Source: CAD feature listing. Evaluate the final solid. Frame: model axes, mm. Give positions to 0.01 mm unless a question says otherwise; leave off trailing zeros. Order: outer loops, then holes, each group sorted by start corner. A loop starts at its lowest first (then second) coordinate and runs counter-clockwise, first axis right, second up. Notation, with made-up numbers: (-10.75, -18) - (26.25, -18) arc R24 cw to (26.25, 17) - close; hole circle Ø4 at (48.5, -32). An arc over 180 degrees is marked (long way). Answer as CSV lines item,"result".
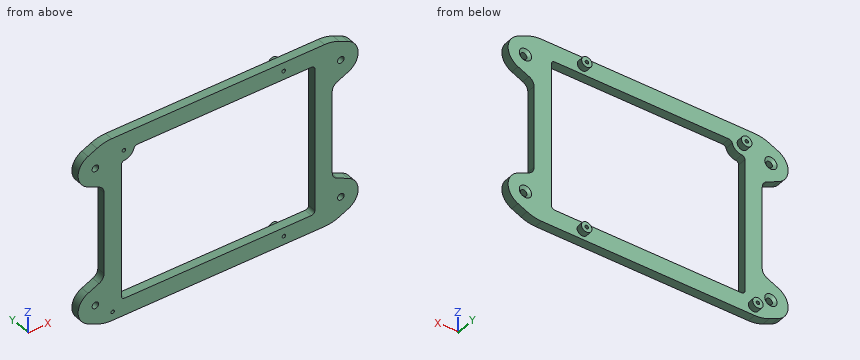
```python
from build123d import *

# Parameters (mm, degrees)
QUARTER_BASE_DEPTH                 = 5
CORNER_SCREW_EXPANSION_SKETCH_R    = 6.025
CORNER_SCREW_EXPANSION_DEPTH       = 5
STANDOFFS_EXTRUSION_SKETCH_R       = 3.025
STANDOFFS_EXTRUSION_DEPTH          = 3.5
SMOOTHIEBOARD_SCREW_HOLES_SKETCH_R = 1.025
SMOOTHIEBOARD_SCREW_HOLES_DEPTH    = 98.695404319
NO_6_MOUNTING_SCREWS_D             = 3.7973
NO_6_MOUNTING_SCREWS_CSINK_D       = 7.0866
NO_6_MOUNTING_SCREWS_CSINK_ANGLE   = 100
INSIDE_CORNER_FILLETS_R            = 2
OUTSIDE_CORNER_FILLETS_1_R         = 5
OUTSIDE_CORNER_FILLETS_2_R         = 20


with BuildPart() as part:
    # Quarter Base Sketch → Quarter Base (new body)
    with BuildSketch(Plane(origin=(0, 0, 0), x_dir=(1, 0, 0), z_dir=(0, 1, 0))):
        with BuildLine():
            Line((0, 53.955), (-66, 53.955))
            Line((-66, 53.955), (-75.226182617, 49.65276039))
            ThreePointArc((-75.226182617, 49.65276039), (-81, 40.58968252), (-75.226182617, 31.526604649))
            Line((-75.226182617, 31.526604649), (-66, 27.224365039))
            Line((-66, 27.224365039), (-66, 0))
            Line((-66, 0), (-56, 0))
            Line((-56, 0), (-56, 43.955))
            Line((-56, 43.955), (0, 43.955))
            Line((0, 43.955), (0, 53.955))
        make_face()
    extrude(amount=QUARTER_BASE_DEPTH)

    # Base Mirror 1: part across plane


with BuildPart() as part_1:
    add(part.part)
    add(part.part.mirror(Plane(origin=(-66, 5, 0), x_dir=(1, 0, 0), z_dir=(0, 0, -1))))

    # Base Mirror 2: part across plane


with BuildPart() as part_2:
    add(part_1.part)
    add(part_1.part.mirror(Plane(origin=(0, 5, -43.955), x_dir=(0, 0, 1), z_dir=(-1, 0, 0))))

    # Corner Screw Expansion Sketch → Corner Screw Expansion (add)
    with BuildSketch(Plane(origin=(0, 5, 0), x_dir=(1, 0, 0), z_dir=(0, 1, 0))):
        with Locations((-54.523, -43.876)):
            Circle(CORNER_SCREW_EXPANSION_SKETCH_R)
    extrude(amount=-CORNER_SCREW_EXPANSION_DEPTH)

    # Standoffs Extrusion Sketch → Standoffs Extrusion (add)
    with BuildSketch(Plane(origin=(0, 5, 0), x_dir=(1, 0, 0), z_dir=(0, 1, 0))):
        with Locations(Location((-61, 48.955, 0), (0, 0, 270))):
            Circle(STANDOFFS_EXTRUSION_SKETCH_R)
        with Locations(Location((-54.523, -43.876, 0), (0, 0, 270))):
            Circle(STANDOFFS_EXTRUSION_SKETCH_R)
        with Locations(Location((37.933, -48.955, 0), (0, 0, 270))):
            Circle(STANDOFFS_EXTRUSION_SKETCH_R)
        with Locations(Location((38.06, 48.955, 0), (0, 0, 270))):
            Circle(STANDOFFS_EXTRUSION_SKETCH_R)
    extrude(amount=STANDOFFS_EXTRUSION_DEPTH)

    # Smoothieboard Screw Holes Sketch → Smoothieboard Screw Holes (cut, through all)
    with BuildSketch(Plane(origin=(0, 8.5, 0), x_dir=(1, 0, 0), z_dir=(0, 1, 0))):
        with Locations(Location((-54.523, -43.876, 0), (0, 0, 270))):
            Circle(SMOOTHIEBOARD_SCREW_HOLES_SKETCH_R)
        with Locations(Location((37.933, -48.955, 0), (0, 0, 270))):
            Circle(SMOOTHIEBOARD_SCREW_HOLES_SKETCH_R)
        with Locations(Location((38.06, 48.955, 0), (0, 0, 270))):
            Circle(SMOOTHIEBOARD_SCREW_HOLES_SKETCH_R)
        with Locations(Location((-61, 48.955, 0), (0, 0, 270))):
            Circle(SMOOTHIEBOARD_SCREW_HOLES_SKETCH_R)
    extrude(amount=-SMOOTHIEBOARD_SCREW_HOLES_DEPTH, mode=Mode.SUBTRACT)

    # No. 6 Mounting Screws (through all)
    with Locations(Plane(origin=(-71, 5, -40.58968252), x_dir=(0, 0, 1), z_dir=(0, 1, 0))):
        with Locations((0, 0), (81.17936504, 0), (81.17936504, 142), (0, 142)):
            CounterSinkHole(NO_6_MOUNTING_SCREWS_D / 2, NO_6_MOUNTING_SCREWS_CSINK_D / 2, counter_sink_angle=NO_6_MOUNTING_SCREWS_CSINK_ANGLE)

    # Inside Corner Fillets
    inside_corner_fillets_edges = [part_2.edges().sort_by_distance(p)[0] for p in [
        (-56, 2.5, -43.955),
        (56, 2.5, -43.955),
        (56, 2.5, 43.955),
        (-48.498517948, 2.5, 43.955),
        (-56, 2.5, 38.034844635),
    ]]
    fillet(inside_corner_fillets_edges, radius=INSIDE_CORNER_FILLETS_R)

    # Outside Corner Fillets 1
    outside_corner_fillets_1_edges = [part_2.edges().sort_by_distance(p)[0] for p in [
        (-66, 2.5, -27.224365039),
        (-66, 2.5, 27.224365039),
        (66, 2.5, -27.224365039),
        (66, 2.5, 27.224365039),
    ]]
    fillet(outside_corner_fillets_1_edges, radius=OUTSIDE_CORNER_FILLETS_1_R)

    # Outside Corner Fillets 2
    outside_corner_fillets_2_edges = [part_2.edges().sort_by_distance(p)[0] for p in [
        (-66, 2.5, -53.955),
        (-66, 2.5, 53.955),
        (66, 2.5, -53.955),
        (66, 2.5, 53.955),
    ]]
    fillet(outside_corner_fillets_2_edges, radius=OUTSIDE_CORNER_FILLETS_2_R)


solid = part_2.part
```
(1) Ray query, line 1 (X direction, y = 1.75, z = 23.5); line 2 (Z direction, x = 71, y = 2.5); line 3 (Z direction, x = -2, y = 3) (3 decimals). Return the intervals inside material, ascending. Write a range as from..to.
Completed:
line 1,"-66..-56, 56..66"
line 2,"-51.62..-42.49, -38.69..-29.56, 29.56..38.69, 42.49..51.62"
line 3,"-53.955..-43.955, 43.955..53.955"
(2) Cut plane A-A (x = -30). Return loops of the section in (y, z) (3 decimals).
Completed:
outline,"(0, -53.955) - (5, -53.955) - (5, -43.955) - (0, -43.955) - close; (0, 43.955) - (5, 43.955) - (5, 53.955) - (0, 53.955) - close"
(3) Contact query for flat-ended pins moving along their axis: pin 1 (2.5 mm diameter, centred on x = -54.523, z = 43.876, fed in from +Y); pin 2 (1.2 mm diameter, centred on x = -61, z = -48.955, fed in from -Y); pin 3 (4.5 mm diameter, centred on x = 71, z = 40.59, fed in from +Y); pin 4 (1.5 mm diameter, centred on y = 2.5, z = 4.5, fed in from +X). Output: stop coordinate, or through.
Completed:
pin 1,"y = 8.5"
pin 2,"through"
pin 3,"y = 3.92"
pin 4,"x = 66"
(4) Cut plane B-B (z = 12.5). Return loops of the section in (x, y), then the cut area to 3 significant figures.
Completed:
outline,"(-66, 0) - (-56, 0) - (-56, 5) - (-66, 5) - close; (56, 0) - (66, 0) - (66, 5) - (56, 5) - close"
area,"100 mm²"
